```python
from build123d import *

# Parameters (mm, degrees)
F0_W     = 85.0682780147
F0_H     = 90.5551686883
F1_DEPTH = 50.8
F3_DEPTH = 90.5561686883
F5_D     = 25.4
F7_W     = 32.6359942555
F7_H     = 14.9547737092
F6_W     = 73.0053722694
F6_H     = 15.5514590442
F8_DEPTH = 25.4


with BuildPart() as f1:
    # F0 (on Top) → F1 (new body)
    with BuildSketch(Plane.XY):
        Rectangle(F0_W, F0_H)
    extrude(amount=F1_DEPTH)

    # F2 (on face) → F3 (cut, through all)
    with BuildSketch(Plane.XZ.offset(45.2775843441)):
        Polygon((42.5341390073, 0), (42.5341390073, 50.8), (-9.8981447518, 50.8), align=None)
    extrude(amount=-F3_DEPTH, mode=Mode.SUBTRACT)

    # F5 (through all)
    with Locations(Plane(origin=(20.594698145, 0, 21.2564381313), x_dir=(0.7181976083, 0, -0.6958392023), z_dir=(0.6958392023, 0, 0.7181976083))):
        with Locations((-13.2798599079, -15.1163674891)):
            Hole(F5_D / 2)

    # F7 (on face) + F6 (on face) → F8 (join)
    with BuildSketch(Plane.XY.offset(50.8)):
        with Locations((-26.2161418796, 37.8001974896)):
            Rectangle(F7_W, F7_H)
    with BuildSketch(Plane(origin=(20.594698145, 0, 21.2564381313), x_dir=(0.7181976083, 0, -0.6958392023), z_dir=(0.6958392023, 0, 0.7181976083))):
        with Locations((-5.9547692273, 37.501854822)):
            Rectangle(F6_W, F6_H)
    extrude(amount=F8_DEPTH, dir=(0, 0, 1))


solid = f1.part
```
The listing builds one solid part. Answer for the finished solid, in the listing's coordinates (mm). A direction names the side the tool comes from. Give positions to 0.01 mm unless a question says otherwise; leave off trailing zeros. Order: outer loops, then holes, each group sorted by start corner. A loop starts at its lowest first (then second) coordinate and runs counter-clockwise, first axis right, second up.
Item 1: Find the intervals of material crossed by probe 1 along Z at (x, y) = (-16.5, -30); probe 2 along Y at (x, z) = (17.5, 26); probe 3 along Y at (x, z) = (-4, 28), in increasing order.
From the geometry:
probe 1: z = 0 to 50.8
probe 2: y = 29.73 to 45.28
probe 3: y = -45.28 to -24, -6.23 to 45.28
Item 2: Given pin 1 Ø12 at (x, y) = (-6, -19) entering from +Z; pin 2 Ø1.5 at (y, z) = (5.5, 23) entering from +X; pin 3 Ø1 at (y, z) = (-13, 43.5) entering from +X, each flat-ended and moving along its own axis, determine where each tip first touches the part or whether it passes through.
From the geometry:
pin 1: stops at z = 50.8
pin 2: stops at x = 19.57
pin 3: stops at x = -1.85
Item 3: The part is cut by section C-C, the plane x = 33.5. Give the vertices of the cut face in (y, z), and give its area (3 significant figures).
From the geometry:
outline: (-45.28, 0) - (45.28, 0) - (45.28, 34.15) - (29.73, 34.15) - (29.73, 8.75) - (-45.28, 8.75) - close
area: 1,190 mm2
Item 4: The part is cut by section B-B, the plane z = 54.5. Give the vertices of the cut face in (x, y).
From the geometry:
outline: (-42.53, 30.32) - (-9.9, 30.32) - (-9.9, 29.73) - (12.5, 29.73) - (12.5, 45.28) - (-42.53, 45.28) - close
Item 5: Which of the six approach directions +Z, -Z, +X, -X, +Y, -Y give full straight-line access (tool end or side, diameter ignored) to faces 4 (the face through (16, 29.726, 38)), 5 (the face through (-26, 30.323, 63)), 6 (the face through (-26, 38, 76.2))?
From the geometry:
face 4: +Z, +X, -Y
face 5: +Z, -X, -Y
face 6: +Z, +X, -X, +Y, -Y
Item 6: The part is cut by section A-A, the plane y = -5. Give the vertices of the cut face in (x, z), and give its area (3 significant figures).
From the geometry:
outline: (-42.53, 0) - (-29.18, 0) - (5.54, 35.84) - (-9.9, 50.8) - (-42.53, 50.8) - close; (-7.8, 0) - (42.53, 0) - (16.57, 25.15) - close
area: 2,340 mm2
Item 7: For a pull along X with two mould halves and no side action, classify faces 1 (the face through (-10, 45.278, 29)), 2 (the face through (21.78, -8.3, 20.11)), 3 (the face through (-12.73, -11.302, 23.354)) as pulls with the +X half, pulls with the -X half, needs draft (parallel to the pull), parting line crosses it, or undercut.
From the geometry:
face 1: needs draft
face 2: pulls with the +X half
face 3: undercut
